Autodesk Inventor part; units mm, degrees
ref_plane "YZ Plane" through (0, 0, 0) normal (1, 0, 0) x (0, 1, 0)
ref_plane "XZ Plane" through (0, 0, 0) normal (0, 1, 0) x (-1, 0, 0)
ref_plane "XY Plane" through (0, 0, 0) normal (0, 0, 1) x (1, 0, 0)
sketch "Sketch6" plane through (0, 0, 0) normal (0, 1, 0) x (-1, 0, 0)
  arc A0 (0, -12.3) -> (0, 12.3) centre (-5.974, 0) ccw
  line L0 (0, -23.7314) -> (0, 23.4378)
  line L1 (0, 12.3) -> (-9.2, 12.3)
  line L2 (0, -12.3) -> (-9.2, -12.3)
  line L3 (-9.2, 12.3) -> (-16, 9.5)
  line L4 (-9.2, -12.3) -> (-16, -9.5)
  line L5 (-16, 9.5) -> (-23.1, 6.8)
  line L6 (-16, -9.5) -> (-23.1, -6.8)
  arc A1 (-23.1, 6.8) -> (-23.1, -6.8) centre (-12.54, 0) ccw
  line L7 (9.3004, 16.6993) -> (-26.9762, 16.6993)
  line L8 (-26.9762, 16.6993) -> (-26.9762, -16.993)
  line L9 (-26.9762, -16.993) -> (9.3004, -16.993)
  line L10 (9.3004, -16.993) -> (9.3004, 16.6993)
  point P0 (0, 0)
  point P1 (7.7, 0)
  point P2 (-25.1, 0)
  dimension "d4" = 0
  dimension "d6" = 0
  dimension "d7" = 7.7
  dimension "d8" = 9.2
  dimension "d9" = 9.2
  dimension "d10" = 2.8
  dimension "d11" = 2.8
  dimension "d12" = 6.8
  dimension "d13" = 6.8
  dimension "d15" = 24.6
  dimension "d16" = 7.1
  dimension "d17" = 7.1
  dimension "d18" = 2.7
  dimension "d19" = 2.7
  dimension "d20" = 2
extrude "Extrusion1" add sketch "Sketch6" along normal blind 10 contours A0 L0 L7 L10 L9 | L0 L9 L8 L7 L1 L3 L5 A1 L6 L4 L2
fillet "Fillet1" radius 2 8 edges at (0, 5, -12.3) (9.2, 5, -12.3) (16, 5, -9.5) (23.1, 5, -6.8) (23.1, 5, 6.8) (16, 5, 9.5) (9.2, 5, 12.3) (0, 5, 12.3)
fillet "Fillet2" radius 2 4 edges at (26.9762, 5, -16.993) (-9.3004, 5, -16.993) (-9.3004, 5, 16.6993) (26.9762, 5, 16.6993)
fillet "Fillet3" radius 0.5 8 edges at (26.3904, 10, -16.4072) (8.8379, 10, -16.993) (-8.7146, 10, -16.4072) (-9.3004, 10, -0.1468) (-8.7146, 10, 16.1135) (8.8379, 10, 16.6993) (26.3904, 10, 16.1135) (26.9762, 10, -0.1468)
fillet "Fillet4" radius 0.5 14 edges at (-0.006, 10, -12.2403) (4.6418, 10, -12.3) (9.1925, 10, -12.262) (12.7829, 10, -10.8247) (23.0498, 10, -6.6911) (19.2278, 10, -8.2725) (25.1, 10, 0) (23.0498, 10, 6.6911) (19.2278, 10, 8.2725) (9.1925, 10, 12.262) (12.7829, 10, 10.8247) (4.6418, 10, 12.3) (-0.006, 10, 12.2403) (-7.7, 10, 0)
properties part number "PipetteProfile_3DPrint"
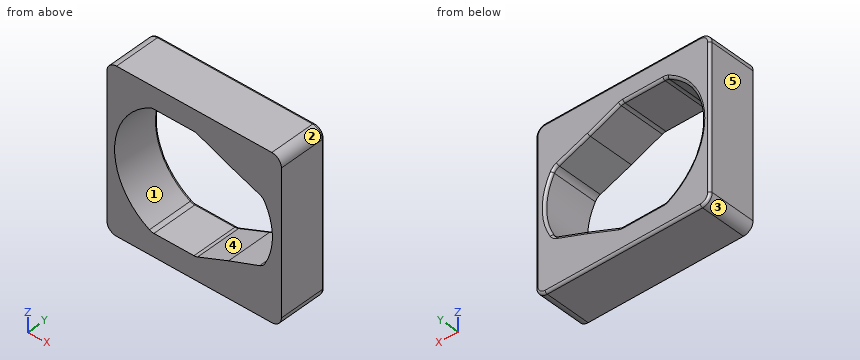
Input: part model. Units: mm. Frame: model coordinates. Face numbers are marked on the shaded views. A direction names the side the tool comes from. Round coordinates to 2 decimals unless told otherwise and drop trailing zeros. Loops run counter-clockwise (first coordinate to the right, second up) from the corner with the lowest first, then second, coordinate; pieces in that order, holes last. Notation, with made-up numbers: (-39, 1.5) -> (-1, 1.5) arc R31 cw to (-1, 29.5) -> close; hole circle Ø10 at (55, -2.5). An arc over 180 degrees is marked (long way). Answer as a JSON object with one key per item and string values. Group by question number.
1) Ray query, L1, parallel to Z at x = 3, y = 7.5; L2, parallel to Z at x = 12.5, y = 5.25; L3, parallel to X at y = 2, z = -10.5. Return the intervals inside material, ascending.
2) Reachability of the marked faces 1 and 2 from +Z, -Z, +X, -X, +Y, -Y: full face, straight path, thin tool, end or side. Return the list, or none.
3) Section query B-B on y = 6.75. Output: boundary loops of the cut face in (x, z), plus the area to 3 significant figures.
4) Draft query along Z for the marked faces 3, 4 and 5. Return one class per face: +Z half, -Z half, draft (parallel to the pull), parting line (faces both ways), or undercut.
5) Section query A-A on x = 5. Output: boundary loops of the cut face in (y, z).
Reply:
{
 "1": {"L1": "z = -16.99 to -12.3, 12.3 to 16.7", "L2": "z = -16.99 to -10.94, 10.94 to 16.7", "L3": "x = -9.3 to -2.79, 13.57 to 26.98"},
 "2": {"face 1": "+Y, -Y", "face 2": "+Z, +X, +Y, -Y"},
 "3": {"outline": "(-9.3, -14.99) arc R2 ccw to (-7.3, -16.99) -> (24.98, -16.99) arc R2 ccw to (26.98, -14.99) -> (26.98, 14.7) arc R2 ccw to (24.98, 16.7) -> (-7.3, 16.7) arc R2 ccw to (-9.3, 14.7) -> close; hole (-0.46, -12.06) arc R2 ccw to (0.48, -12.3) -> (8.8, -12.3) arc R2 ccw to (9.57, -12.15) -> (16, -9.5) -> (22.46, -7.05) arc R2 ccw to (23.49, -6.16) arc R12.56 ccw to (23.49, 6.16) arc R2 ccw to (22.46, 7.05) -> (16, 9.5) -> (9.57, 12.15) arc R2 ccw to (8.8, 12.3) -> (0.48, 12.3) arc R2 ccw to (-0.46, 12.06) arc R13.67 ccw to start", "area": "575 mm2"},
 "4": {"face 3": "-Z half", "face 4": "undercut", "face 5": "draft"},
 "5": {"outline": "(0, -16.99) -> (9.5, -16.99) arc R0.5 ccw to (10, -16.49) -> (10, -12.8) arc R0.5 ccw to (9.5, -12.3) -> (0, -12.3) -> close; (0, 12.3) -> (9.5, 12.3) arc R0.5 ccw to (10, 12.8) -> (10, 16.2) arc R0.5 ccw to (9.5, 16.7) -> (0, 16.7) -> close"}
}
